Part model, mm, in its own coordinate system. Give positions to 0.01 mm unless a question says otherwise; leave off trailing zeros. Write each loop counter-clockwise with the first axis right and the second up, starting at its lowest first coordinate (ties: lowest second). Pieces come first, ordered by that corner, then holes. Notation, with made-up numbers: M 28.5,-33 L 80.5,-33 A13 ccw 80.5,-18 Z; hole C 67.5,53.5 d2. An arc over 180 degrees is marked long. Use a Markdown table: item, result.
```python
from build123d import *

# Parameters (mm, degrees)
SALIENTE_EXTRUIR1_DEPTH = 5
CROQUIS2_R              = 14
CROQUIS2_R_2            = 12.5
CORTAR_EXTRUIR1_DEPTH   = 5


with BuildPart() as part:
    # Croquis1 → Saliente-Extruir1 (new body)
    with BuildSketch(Plane.XY):
        with BuildLine():
            Line((5, 0), (370, 0))
            ThreePointArc((370, 0), (400, 30), (370, 60))
            Line((370, 60), (5, 60))
            ThreePointArc((5, 60), (1.464466094, 58.535533906), (0, 55))
            Line((0, 55), (0, 5))
            ThreePointArc((0, 5), (1.464466094, 1.464466094), (5, 0))
        make_face()
    extrude(amount=SALIENTE_EXTRUIR1_DEPTH)

    # Croquis2 → Cortar-Extruir1 (cut)
    with BuildSketch(Plane.XY.offset(5)):
        with Locations((370, 30)):
            Circle(CROQUIS2_R)
        with Locations((35, 30)):
            Circle(CROQUIS2_R_2)
        with Locations((70, 30)):
            Circle(CROQUIS2_R)
    extrude(amount=-CORTAR_EXTRUIR1_DEPTH, mode=Mode.SUBTRACT)


solid = part.part
```
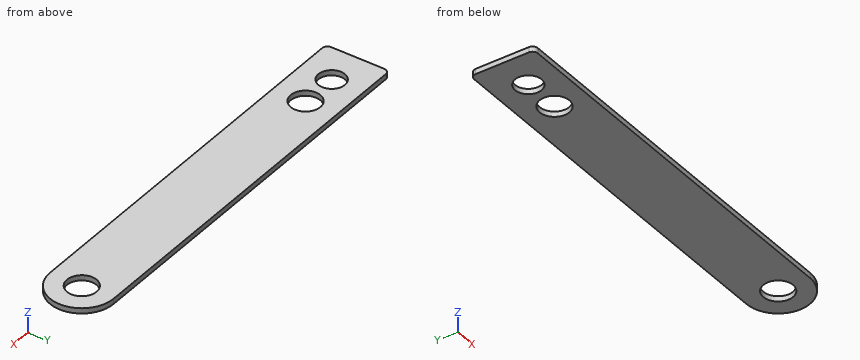
1. Cut at A-A, the plane y = 30. Give the cut face in (x, z), then the cut area to 4 significant figures.
Findings below:
| item | result |
|---|---|
| outline | M 0,0 L 22.5,0 L 22.5,5 L 0,5 Z; M 47.5,0 L 56,0 L 56,5 L 47.5,5 Z; M 84,0 L 356,0 L 356,5 L 84,5 Z; M 384,0 L 400,0 L 400,5 L 384,5 Z |
| area | 1,595 mm2 |
2. Cut at C-C, the plane z = 1.8. Give the cut face in (x, y).
Findings below:
| item | result |
|---|---|
| outline | M 0,5 A5 ccw 5,0 L 370,0 A30 ccw 370,60 L 5,60 A5 ccw 0,55 Z; hole C 35,30 d25; hole C 70,30 d28; hole C 370,30 d28 |
3. Cut at B-B, the plane x = 70. Give the cut face in (y, z), then the cut area to 3 significant figures.
Findings below:
| item | result |
|---|---|
| outline | M 0,0 L 16,0 L 16,5 L 0,5 Z; M 44,0 L 60,0 L 60,5 L 44,5 Z |
| area | 160 mm2 |
4. Drill centre lines: L1, parallel to Y at x = 370, z = 2.4; L2, parallel to X at y = 24, z = 4.4; L3, parallel to X at y = 34.5, z = 4. Where is each one in solid material? Low to high.
Findings below:
| item | result |
|---|---|
| L1 | 0 to 16, 44 to 60 |
| L2 | 0 to 24.03, 45.97 to 57.35, 82.65 to 357.35, 382.65 to 399.39 |
| L3 | 0 to 23.34, 46.66 to 56.74, 83.26 to 356.74, 383.26 to 399.66 |
